Verification items for the finished model (mm, model axes). Face numbers are marked on the shaded views. Coordinates: 2 decimals unless noted, no trailing zeros. Order: outer loops, then holes, each group sorted by start corner. A loop starts at its lowest first (then second) coordinate and runs counter-clockwise, first axis right, second up. Notation, with made-up numbers: M 13.5,63.25 L 19.5,63.25 A13 ccw 19.5,84.25 Z; hole C 26.25,19 d7. An arc over 180 degrees is marked long. Answer as a JSON object with one key per item and string values. Group by question number.
(1) Mould release check, pull along Z, two halves, no side actions. Record for the marked faces 1, 2 and 3: released by +Z, released by -Z, zero draft, split by the parting line, or undercut.
(2) Cross-section at A-A (y = -31). Enter the section's corners in (x, z).
(3) Gauge pin test, flat ends, axial feed: pin 1 Ø1.2 at (y, z) = (-6.5, 37) entering from -X; pin 2 Ø3.5 at (x, y) = (59.45, 0.5) entering from -Z; pin 3 Ø1.2 at (y, z) = (-8.5, 36) entering from +X. Record the tip position at first contact, or that the pin passes through.
(4) Cross-section at B-B (x = -19). Enter the section's corners in (y, z).
(5) Cross-section at C-C (z = 30.5). Enter the section's corners in (x, y), plus the area to 3 significant figures.
(6) Material ranges on line 1 (Y direction, x = 59.45, z = 30.25); line 2 (Z direction, x = 7.5, y = -19); line 3 (X direction, y = -2.5, z = -30), recorded low to high.
(7) Cross-section at D-D (z = 17). Enter the section's corners in (x, y), plus the area to 3 significant figures.
from build123d import *

# Parameters (mm, degrees)
BOSS_EXTRUDE1_DEPTH             = 4
SKETCH3_W                       = 7.1
SKETCH3_H                       = 8
BOSS_EXTRUDE3_DEPTH             = 3
SKETCH4_R                       = 2.05
CUT_EXTRUDE1_DEPTH              = 7
MIRROR2_COPY_1_SKETCH_W         = 7.1
MIRROR2_COPY_1_SKETCH_H         = 8
MIRROR2_COPY_1_DEPTH            = 3
MIRROR2_COPY_2_SKETCH_R         = 2.05
MIRROR2_COPY_2_DEPTH            = 7
SKETCH5_W                       = 60
SKETCH5_H                       = 9
CUT_EXTRUDE2_DEPTH              = 75.953318806
FILLET1_R                       = 2
SKETCH7_W                       = 111.8
SKETCH7_H                       = 1
CUT_EXTRUDE3_DEPTH              = 75.953318806
SKETCH8_W                       = 126
SKETCH8_H                       = 2
BOSS_EXTRUDE4_DEPTH             = 38
SKETCH9_W                       = 12
SKETCH9_H                       = 18
CUT_EXTRUDE4_DEPTH              = 10
SKETCH10_W                      = 7.1
SKETCH10_H                      = 4
BOSS_EXTRUDE5_DEPTH             = 3
SKETCH12_W                      = 1.5
SKETCH12_H                      = 4
BOSS_EXTRUDE6_DEPTH             = 2
SKETCH13_W                      = 40
SKETCH13_H                      = 2
BOSS_EXTRUDE7_DEPTH             = 38
SKETCH14_W                      = 1.5
SKETCH14_H                      = 4
BOSS_EXTRUDE8_DEPTH             = 1
BOSS_EXTRUDE9_REACH             = 85.271
BOSS_EXTRUDE9_DIRECTION_2_REACH = 85.271
SKETCH16_W                      = 20
SKETCH16_H                      = 14
SKETCH16_W_2                    = 14.5
SKETCH16_H_2                    = 9
BOSS_EXTRUDE10_DEPTH            = 4
SKETCH17_W                      = 12
SKETCH17_H                      = 18
CUT_EXTRUDE5_DEPTH              = 84.270643086
SKETCH18_W                      = 6
SKETCH18_H                      = 6
CUT_EXTRUDE6_DEPTH              = 86.170417399
SKETCH22_R                      = 1.25
CUT_EXTRUDE7_DEPTH              = 4
SKETCH25_W                      = 6
SKETCH25_H                      = 38
CUT_EXTRUDE11_DEPTH             = 10
CUT_EXTRUDE12_DEPTH             = 85.029756634
CUT_EXTRUDE12_DEPTH_BACK        = 85.029756634
SKETCH26_W                      = 5.701552738
SKETCH26_H                      = 30.562488548
SKETCH26_W_2                    = 7.53419365
SKETCH26_H_2                    = 28.524331859
SKETCH27_R                      = 1.25
CUT_EXTRUDE13_DEPTH             = 86.170417399


with BuildPart() as part:
    # Sketch1 → Boss-Extrude1 (new body)
    with BuildSketch(Plane(origin=(0, 0, 0), x_dir=(1, 0, 0), z_dir=(0, 1, 0))):
        Polygon((-63, -33), (-55.9, -33), (-55.9, -40), (55.9, -40), (55.9, -33), (63, -33), (63, 33), (55.9, 33), (55.9, 40), (-55.9, 40), (-55.9, 33), (-63, 33), align=None)
    extrude(amount=BOSS_EXTRUDE1_DEPTH)

    # Sketch3 → Boss-Extrude3 (add)
    with BuildSketch(Plane.XZ):
        with Locations((-59.45, -29)):
            Rectangle(SKETCH3_W, SKETCH3_H)
    boss_extrude3 = extrude(amount=BOSS_EXTRUDE3_DEPTH)

    # Sketch4 → Cut-Extrude1 (cut)
    with BuildSketch(Plane(origin=(0, 0, -33), x_dir=(-1, 0, 0), z_dir=(0, 0, -1))):
        with Locations((59.45, 0.5)):
            Circle(SKETCH4_R)
    cut_extrude1 = extrude(amount=-CUT_EXTRUDE1_DEPTH, mode=Mode.SUBTRACT)

    # Mirror1: Boss-Extrude3, Cut-Extrude1 across plane
    add(boss_extrude3.mirror(Plane(origin=(0, 0, 0), x_dir=(0, 0, 1), z_dir=(1, 0, 0))))
    add(cut_extrude1.mirror(Plane(origin=(0, 0, 0), x_dir=(0, 0, 1), z_dir=(1, 0, 0))), mode=Mode.SUBTRACT)

    # Mirror2: Boss-Extrude3, Cut-Extrude1 across plane
    add(boss_extrude3.mirror(Plane.XY))
    add(cut_extrude1.mirror(Plane.XY), mode=Mode.SUBTRACT)

    # Mirror2 copy 1 sketch → Mirror2 copy 1 (add)
    with BuildSketch(Plane(origin=(0, 0, 0), x_dir=(-1, 0, 0), z_dir=(0, -1, 0))):
        with Locations((-59.45, -29)):
            Rectangle(MIRROR2_COPY_1_SKETCH_W, MIRROR2_COPY_1_SKETCH_H)
    extrude(amount=MIRROR2_COPY_1_DEPTH)

    # Mirror2 copy 2 sketch → Mirror2 copy 2 (cut)
    with BuildSketch(Plane.XY.offset(33)):
        with Locations((59.45, 0.5)):
            Circle(MIRROR2_COPY_2_SKETCH_R)
    extrude(amount=-MIRROR2_COPY_2_DEPTH, mode=Mode.SUBTRACT)

    # Sketch5 → Cut-Extrude2 (cut, through all)
    with BuildSketch(Plane(origin=(0, 4, 0), x_dir=(1, 0, 0), z_dir=(0, 1, 0))):
        with Locations((0, 33.5)):
            Rectangle(SKETCH5_W, SKETCH5_H)
    extrude(amount=-CUT_EXTRUDE2_DEPTH, mode=Mode.SUBTRACT)

    # Fillet1
    fillet1_edges = [part.edges().sort_by_distance(p)[0] for p in [
        (-30, 2, -29),
        (-30, 2, -38),
        (30, 2, -38),
        (30, 2, -29),
    ]]
    fillet(fillet1_edges, radius=FILLET1_R)

    # Sketch7 → Cut-Extrude3 (cut, through all)
    with BuildSketch(Plane(origin=(0, 4, 0), x_dir=(1, 0, 0), z_dir=(0, 1, 0))):
        with Locations((0, 39.5)):
            Rectangle(SKETCH7_W, SKETCH7_H)
        with Locations((0, -39.5)):
            Rectangle(SKETCH7_W, SKETCH7_H)
    extrude(amount=-CUT_EXTRUDE3_DEPTH, mode=Mode.SUBTRACT)

    # Sketch8 → Boss-Extrude4 (add)
    with BuildSketch(Plane.XZ):
        with Locations((0, 20)):
            Rectangle(SKETCH8_W, SKETCH8_H)
    extrude(amount=BOSS_EXTRUDE4_DEPTH)

    # Sketch9 → Cut-Extrude4 (cut)
    with BuildSketch(Plane(origin=(0, 4, 0), x_dir=(1, 0, 0), z_dir=(0, 1, 0))):
        with Locations((-49.9, -30)):
            Rectangle(SKETCH9_W, SKETCH9_H)
    extrude(amount=-CUT_EXTRUDE4_DEPTH, mode=Mode.SUBTRACT)

    # Sketch10 → Boss-Extrude5 (add)
    with BuildSketch(Plane.XZ.offset(3)):
        with Locations((-59.45, 23)):
            Rectangle(SKETCH10_W, SKETCH10_H)
        with Locations((59.45, 23)):
            Rectangle(SKETCH10_W, SKETCH10_H)
    extrude(amount=-BOSS_EXTRUDE5_DEPTH)

    # Sketch12 → Boss-Extrude6 (add)
    # profile 1 of 2: a face of its own
    with BuildSketch(Plane.ZY.offset(56)):
        Polygon((21, -5.8), (21, -16.2), (23.7, -13.5), (23.7, -8.5), align=None)
        with Locations((22.35, -11)):
            Rectangle(SKETCH12_W, SKETCH12_H, mode=Mode.SUBTRACT)
    # profile 2 of 2: a face of its own
    with BuildSketch(Plane.ZY.offset(56)):
        Polygon((21, -20.8), (21, -31.2), (23.7, -28.5), (23.7, -23.5), align=None)
        with Locations((22.35, -26)):
            Rectangle(SKETCH12_W, SKETCH12_H, mode=Mode.SUBTRACT)
    boss_extrude6 = extrude(amount=-BOSS_EXTRUDE6_DEPTH)

    # Mirror3: Boss-Extrude6 across plane
    add(boss_extrude6.mirror(Plane(origin=(-49.9, 0, 0), x_dir=(0, 0, 1), z_dir=(1, 0, 0))))

    # Sketch13 → Boss-Extrude7 (add)
    with BuildSketch(Plane.XZ):
        with Locations((0, -20.5)):
            Rectangle(SKETCH13_W, SKETCH13_H)
    extrude(amount=BOSS_EXTRUDE7_DEPTH)

    # Sketch14 → Boss-Extrude8 (add, symmetric)
    # profile 1 of 2: a face of its own
    with BuildSketch(Plane(origin=(0, 0, 0), x_dir=(0, 0, -1), z_dir=(1, 0, 0))):
        Polygon((24.2, -8.5), (21.5, -5.8), (21.5, -16.2), (24.2, -13.5), align=None)
        with Locations((22.85, -11)):
            Rectangle(SKETCH14_W, SKETCH14_H, mode=Mode.SUBTRACT)
    # profile 2 of 2: a face of its own
    with BuildSketch(Plane(origin=(0, 0, 0), x_dir=(0, 0, -1), z_dir=(1, 0, 0))):
        Polygon((24.2, -28.5), (24.2, -23.5), (21.5, -20.8), (21.5, -31.2), align=None)
        with Locations((22.85, -26)):
            Rectangle(SKETCH14_W, SKETCH14_H, mode=Mode.SUBTRACT)
    extrude(amount=BOSS_EXTRUDE8_DEPTH, both=True)

    # Boss-Extrude9: up to this face of the body (flat: up to its plane)
    boss_extrude9_end = Plane(part.part.faces().sort_by_distance((-20, -19, -20.5))[0])
    # Sketch15 → Boss-Extrude9 (add, up to the picked face)
    with BuildSketch(Plane(origin=(0, 0, 0), x_dir=(0, 0, -1), z_dir=(1, 0, 0)), mode=Mode.PRIVATE) as boss_extrude9_sk1:
        Polygon((19.5, 0), (19.5, -5), (16.613248654, 0), align=None)
    boss_extrude9_tool1 = split(extrude(boss_extrude9_sk1.sketch, amount=-BOSS_EXTRUDE9_REACH, mode=Mode.PRIVATE), bisect_by=boss_extrude9_end, keep=Keep.BOTH, mode=Mode.PRIVATE)
    add(boss_extrude9_tool1.solids().sort_by(Axis((0, -1.666667, -18.53775), (-1, 0, 0)))[0])

    # Boss-Extrude9 direction 2: up to this face of the body (flat: up to its plane)
    boss_extrude9_direction_2_end = Plane(part.part.faces().sort_by_distance((20, -19, -20.5))[0])
    # Sketch15 → Boss-Extrude9 direction 2 (add, up to the picked face)
    with BuildSketch(Plane(origin=(0, 0, 0), x_dir=(0, 0, -1), z_dir=(1, 0, 0)), mode=Mode.PRIVATE) as boss_extrude9_direction_2_sk1:
        Polygon((19.5, 0), (19.5, -5), (16.613248654, 0), align=None)
    boss_extrude9_direction_2_tool1 = split(extrude(boss_extrude9_direction_2_sk1.sketch, amount=BOSS_EXTRUDE9_DIRECTION_2_REACH, mode=Mode.PRIVATE), bisect_by=boss_extrude9_direction_2_end, keep=Keep.BOTH, mode=Mode.PRIVATE)
    add(boss_extrude9_direction_2_tool1.solids().sort_by(Axis((0, -1.666667, -18.53775), (1, 0, 0)))[0])

    # Sketch16 → Boss-Extrude10 (add)
    with BuildSketch(Plane.XY.offset(39)):
        with Locations((30, -7)):
            Rectangle(SKETCH16_W, SKETCH16_H)
        with Locations((30, -7)):
            Rectangle(SKETCH16_W_2, SKETCH16_H_2, mode=Mode.SUBTRACT)
    extrude(amount=-BOSS_EXTRUDE10_DEPTH)

    # Sketch17 → Cut-Extrude5 (cut, through all)
    with BuildSketch(Plane.XZ):
        with Locations((49.9, 30)):
            Rectangle(SKETCH17_W, SKETCH17_H)
    extrude(amount=-CUT_EXTRUDE5_DEPTH, mode=Mode.SUBTRACT)

    # Sketch18 → Cut-Extrude6 (cut, through all)
    with BuildSketch(Plane(origin=(0, 4, 0), x_dir=(1, 0, 0), z_dir=(0, 1, 0))):
        with Locations((52.9, 36)):
            Rectangle(SKETCH18_W, SKETCH18_H)
        with Locations((-52.9, 36)):
            Rectangle(SKETCH18_W, SKETCH18_H)
    extrude(amount=-CUT_EXTRUDE6_DEPTH, mode=Mode.SUBTRACT)

    # Sketch22 → Cut-Extrude7 (cut)
    with BuildSketch(Plane(origin=(0, 4, 0), x_dir=(1, 0, 0), z_dir=(0, 1, 0))):
        with Locations(Location((31, 25, 0), (0, 0, 270))):
            Circle(SKETCH22_R)
        with Locations(Location((-31, -17, 0), (0, 0, 270))):
            Circle(SKETCH22_R)
    extrude(amount=-CUT_EXTRUDE7_DEPTH, mode=Mode.SUBTRACT)

    # Sketch25 → Cut-Extrude11 (cut)
    with BuildSketch(Plane(origin=(0, 0, -21.5), x_dir=(-1, 0, 0), z_dir=(0, 0, -1))):
        with Locations((-17, -19)):
            Rectangle(SKETCH25_W, SKETCH25_H)
        with Locations((17, -19)):
            Rectangle(SKETCH25_W, SKETCH25_H)
    extrude(amount=-CUT_EXTRUDE11_DEPTH, mode=Mode.SUBTRACT)

    # Sketch26 → Cut-Extrude12 (cut, two sides: drawn at the far end of the back side and taken through both)
    with BuildSketch(Plane.ZY.offset(1).offset(-CUT_EXTRUDE12_DEPTH_BACK)):
        with Locations((-24.350776369, -21.081244274)):
            Rectangle(SKETCH26_W, SKETCH26_H)
        with Locations((24.767096825, -20.06216593)):
            Rectangle(SKETCH26_W_2, SKETCH26_H_2)
    extrude(amount=CUT_EXTRUDE12_DEPTH + CUT_EXTRUDE12_DEPTH_BACK, mode=Mode.SUBTRACT)

    # Sketch27 → Cut-Extrude13 (cut, through all)
    with BuildSketch(Plane(origin=(0, 4, 0), x_dir=(1, 0, 0), z_dir=(0, 1, 0))):
        with Locations(Location((-33.2, 26.5, 0), (0, 0, 270))):
            Circle(SKETCH27_R)
        with Locations(Location((-33.2, -30.5, 0), (0, 0, 270))):
            Circle(SKETCH27_R)
        with Locations(Location((38.8, -30.5, 0), (0, 0, 270))):
            Circle(SKETCH27_R)
        with Locations(Location((38.8, 26.5, 0), (0, 0, 270))):
            Circle(SKETCH27_R)
    extrude(amount=-CUT_EXTRUDE13_DEPTH, mode=Mode.SUBTRACT)


solid = part.part
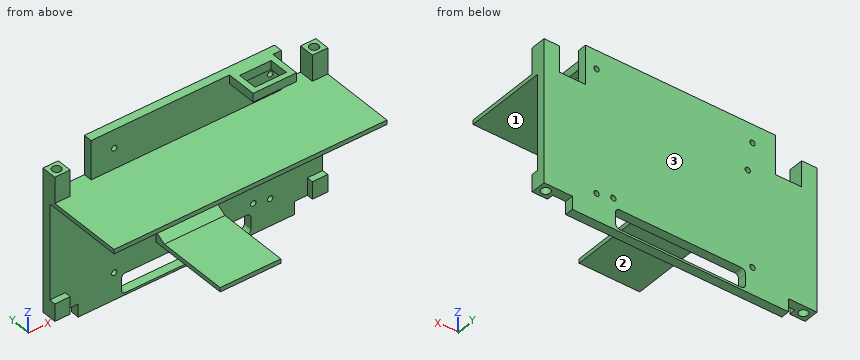
Taken from the geometry:
{
 "1": {"face 1": "undercut", "face 2": "released by -Z", "face 3": "zero draft"},
 "2": {"outline": "M -63,19 L 63,19 L 63,21 L -63,21 Z; M -14,-21.5 L 14,-21.5 L 14,-19.5 L -14,-19.5 Z"},
 "3": {"pin 1": "stops at x = 20", "pin 2": "stops at z = -26", "pin 3": "stops at x = 40"},
 "4": {"outline": "M -38,19 L 0,19 L 0,-29 L 4,-29 L 4,39 L 0,39 L 0,21 L -38,21 Z; M 0,-39 L 4,-39 L 4,-38 L 0,-38 Z"},
 "5": {"outline": "M -63,-3 L -55.9,-3 L -55.9,4 L -63,4 Z; M -43.9,0 L -34.45,0 L -34.45,4 L -43.9,4 Z; M -31.95,0 L 37.55,0 L 37.55,4 L -31.95,4 Z; M 40.05,0 L 43.9,0 L 43.9,4 L 40.05,4 Z; M 55.9,-3 L 63,-3 L 63,4 L 55.9,4 Z; hole C -59.45,0.5 d4.1; hole C 59.45,0.5 d4.1", "area": "404 mm²"},
 "6": {"line 1": "y = -3 to -1.55, 2.55 to 4", "line 2": "z = -21.5 to -19.5, 19 to 21", "line 3": "x = -63 to -55.9, 55.9 to 63"},
 "7": {"outline": "M -63,0 L -32.25,0 L -32.25,4 L -63,4 Z; M -29.75,0 L 63,0 L 63,4 L -29.75,4 Z", "area": "494 mm²"}
}
